Check sheet for the drawn part. Datum: minimum x, y, z corner. Units: mm. Round coordinates to 2 decimals unless told otherwise and drop trailing zeros. Write each loop counter-clockwise with the first axis right and the second up, starting at its lowest first coordinate (ties: lowest second). Pieces come first, ordered by that corner, then holes. Notation, with made-up numbers: M 51.5,78 L 65.5,78 A20 cw 65.5,85 Z; hole C -16.5,53.5 d1. An arc over 180 degrees is marked long. One line per item, written item: value.
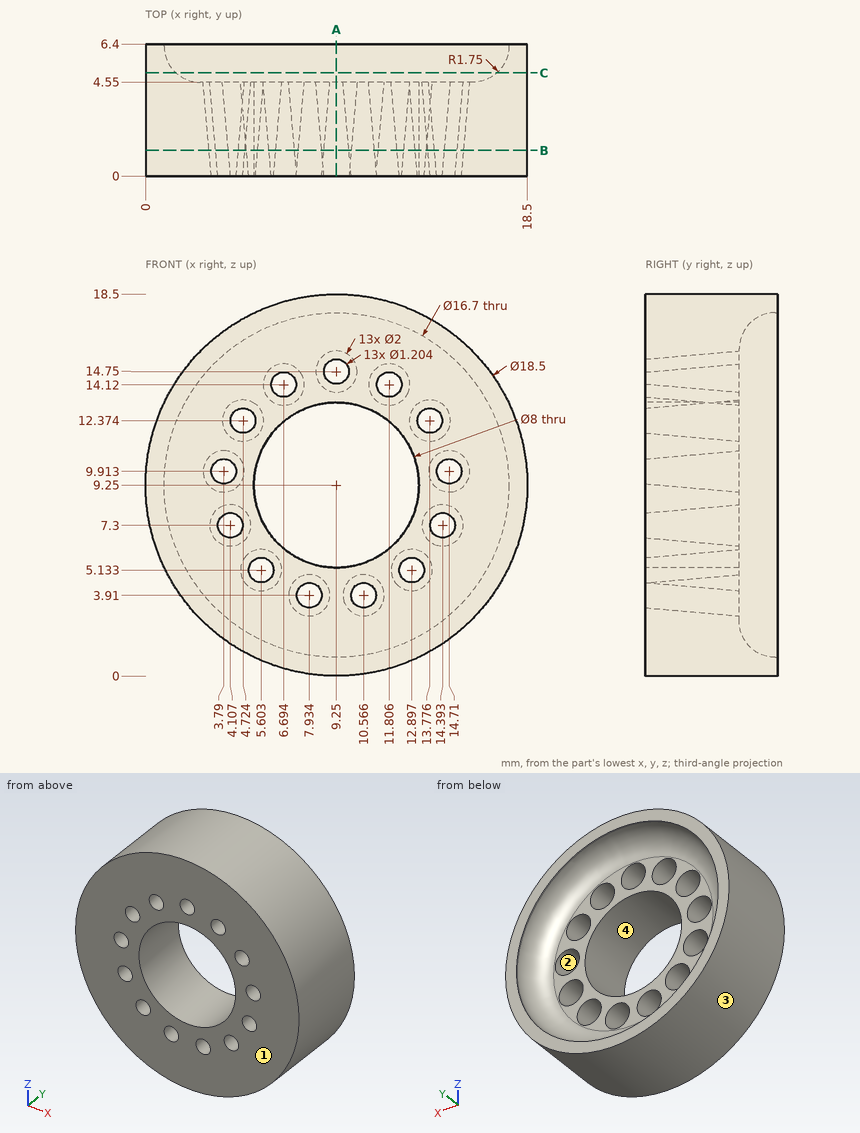
Q1. Depth check by flat-ended pin: P1, Ø1.5, axis at y = 3.5, z = 2, coming from the +X side; P2, Ø3, axis at x = 12.5, z = 10.5, coming from the +Y side; P3, Ø7, axis at x = 9.25, z = 9.25, coming from the +Y side; P4, Ø3, axis at y = 5.5, z = 14, coming from the -X side. Enter the tip coordinate at first touch or a pass-through.
Completed:
P1: x = 15.83
P2: y = 4.55
P3: through
P4: x = 0.59
Q2. Sectioned sample at A-A on x = 9.25. Enter the section's corners in (y, z).
Completed:
outline: M 0,0 L 6.4,0 L 6.4,0.9 L 6.3,0.9 A1.75 cw 4.55,2.65 L 4.55,5.25 L 0,5.25 Z; M 0,13.25 L 4.55,13.25 L 4.55,13.75 L 0,14.15 Z; M 0,15.35 L 4.55,15.75 L 4.55,15.85 A1.75 cw 6.3,17.6 L 6.4,17.6 L 6.4,18.5 L 0,18.5 Z
Q3. Draft check along Z on the marked faces 1, 2, 3 and 4. Enter one of: pulls with the +Z half, pulls with the -Z half, needs draft (parallel to the pull), parting line crosses it, or undercut.
Completed:
face 1: needs draft
face 2: undercut
face 3: parting line crosses it
face 4: undercut
Q4. Sectioned sample at C-C on y = 5. Enter the section's corners in (x, z).
Completed:
outline: C 9.25,9.25 d18.5; hole C 9.25,9.25 d15.54
Q5. Scan lines: line 1 (X direction, y = 3.35, z = 9.25); line 2 (Z direction, x = 8.5, y = 3) (1 decimal); line 3 (Z direction, x = 11.75, y = 3.5) (1 decimal). Record each from-to range of solid material in increasing order. Write a range as [from, to].
Completed:
line 1: [0, 3.19], [4.39, 5.25], [13.25, 14.11], [15.31, 18.5]
line 2: [0, 3.3], [4.6, 5.3], [13.2, 14.3], [15.2, 18.5]
line 3: [0.3, 6.1], [12.4, 13.2], [15, 18.2]
Q6. Sectioned sample at B-B on y = 1.25. State how many separate pieces and enclosed holes the cut face has, and give its area (3 significant figures).
Completed:
separate pieces: 1
enclosed holes: 14
area: 198 mm^2
